```python
from build123d import *

# Parameters (mm, degrees)
F0_W     = 76.2
F0_H     = 76.2
F1_DEPTH = 76.2
F6_R     = 6.35
F6_R_2   = 12.7
F7_DEPTH = 76.2010001
F8_R     = 5.08


with BuildPart() as f1:
    # F0 (on Top) → F1 (new body)
    with BuildSketch(Plane.XY):
        Rectangle(F0_W, F0_H)
    extrude(amount=F1_DEPTH)

    # F2 (on face) → F5 section 0
    with BuildSketch(Plane(origin=(-38.1, 0, 0), x_dir=(0, -1, 0), z_dir=(-1, 0, 0))):
        Polygon((38.1, 34.29), (38.1, 57.15), (27.94, 57.15), (27.94, 63.5), (7.62, 63.5), (7.62, 25.4), (27.94, 25.4), (27.94, 34.29), align=None)
    # F4 (on face) → F5 section 1
    with BuildSketch(Plane.YZ.offset(38.1)):
        Polygon((-27.94, 57.15), (-38.1, 57.15), (-38.1, 20.85388407), (-27.94, 20.85388407), (-27.94, 11.96388407), (-7.62, 11.96388407), (-7.62, 63.5), (-27.94, 63.5), align=None)
    loft(mode=Mode.SUBTRACT)

    # F6 (on face) → F7 (cut, through all)
    with BuildSketch(Plane.XY.offset(76.2)):
        with Locations((-19.05, -17.78)):
            Circle(F6_R)
        with Locations((19.05, -17.78)):
            Circle(F6_R)
        with Locations((0, 17.78)):
            Circle(F6_R_2)
    extrude(amount=-F7_DEPTH, mode=Mode.SUBTRACT)

    # F8
    f8_edges = [f1.edges().sort_by_distance(p)[0] for p in [
        (38.1, 38.1, 38.1),
        (-38.1, 38.1, 38.1),
        (38.1, -38.1, 10.426942),
        (-38.1, -38.1, 17.145),
        (38.1, -38.1, 66.675),
        (-38.1, -38.1, 66.675),
    ]]
    fillet(f8_edges, radius=F8_R)


solid = f1.part
```
Can you work these out from the model? Positions are in its coordinate system, mm. A direction names the side the tool comes from. Round coordinates to 2 decimals unless told otherwise and drop trailing zeros. Order: outer loops, then holes, each group sorted by start corner. A loop starts at its lowest first (then second) coordinate and runs counter-clockwise, first axis right, second up. Notation, with made-up numbers: (70.25, -24.75) -> (85.25, -24.75) arc R26 cw to (85.25, 13.25) -> close; hole circle Ø5 at (-6.5, -15.75). An arc over 180 degrees is marked (long way). Return JSON: item names as keys, results as strings. Group by question number.
1. If we section it at A-A, the plane y = 17.78: Write out the boundary of the cut face in (x, z), then the cut area to 3 significant figures.
2. If we section it at B-B, the plane y = -17.78: Write out the boundary of the cut face in (x, z), then the cut area to 3 significant figures.
3. Which directions (+Z, -Z, +X, -X, +Y, -Y) give clear straight access to the entire face, cutting with the end or side of a thin tool? Please do faces 5 (the face through (1, -18, 63.5)), 6 (the face through (-1, 1, 0)), 7 (the face through (0.53, -32.95, 27.48)).
4. If we section it at C-C, the plane x = 19.05: Count the separate pieces of the cut face and the enclosed holes in it, then the cut area to 3 significant figures.
5. I need wall thicknesses on line 1 (Y direction, x = 19.05, z = 4.25); line 2 (Y direction, x = 3, z = 62.5); line 3 (Y direction, x = 14.5, z = 19). Which ranges of each line are inside material? Lowest first, please. Write a range as [from, to].
6. We'd pull the mould along Y, two halves only. Please class faces 1 (the face through (0.53, -17.64, 18.59)), 2 (the face through (-24.09, -21.64, 69.94)), 3 (the face through (0, -38.1, 13)), 4 (the face through (-38.1, 7, 38)): released by +Y, released by -Y, zero draft, split by the parting line, or undercut.
Output values:
{
 "1": {"outline": "(-38.1, 0) -> (-12.7, 0) -> (-12.7, 76.2) -> (-38.1, 76.2) -> close; (12.7, 0) -> (38.1, 0) -> (38.1, 76.2) -> (12.7, 76.2) -> close", "area": "3,870 mm²"},
 "2": {"outline": "(-38.1, 0) -> (-25.4, 0) -> (-25.4, 23.16) -> (-38.1, 25.4) -> close; (-38.1, 63.5) -> (-25.4, 63.5) -> (-25.4, 76.2) -> (-38.1, 76.2) -> close; (-12.7, 0) -> (12.7, 0) -> (12.7, 16.44) -> (-12.7, 20.92) -> close; (-12.7, 63.5) -> (12.7, 63.5) -> (12.7, 76.2) -> (-12.7, 76.2) -> close; (25.4, 0) -> (38.1, 0) -> (38.1, 11.96) -> (25.4, 14.2) -> close; (25.4, 63.5) -> (38.1, 63.5) -> (38.1, 76.2) -> (25.4, 76.2) -> close", "area": "1,590 mm²"},
 "3": {"face 5": "+X, -X", "face 6": "-Z, +X, -X, +Y, -Y", "face 7": "+X, -Y"},
 "4": {"separate pieces": "3", "enclosed holes": "0", "area": "4,140 mm²"},
 "5": {"line 1": "[-38.1, -24.13], [-11.43, 38.1]", "line 2": "[-38.1, -27.94], [-7.62, 5.44], [30.12, 38.1]", "line 3": "[-38.1, -27.94], [-7.62, 38.1]"},
 "6": {"face 1": "undercut", "face 2": "undercut", "face 3": "released by -Y", "face 4": "zero draft"}
}
